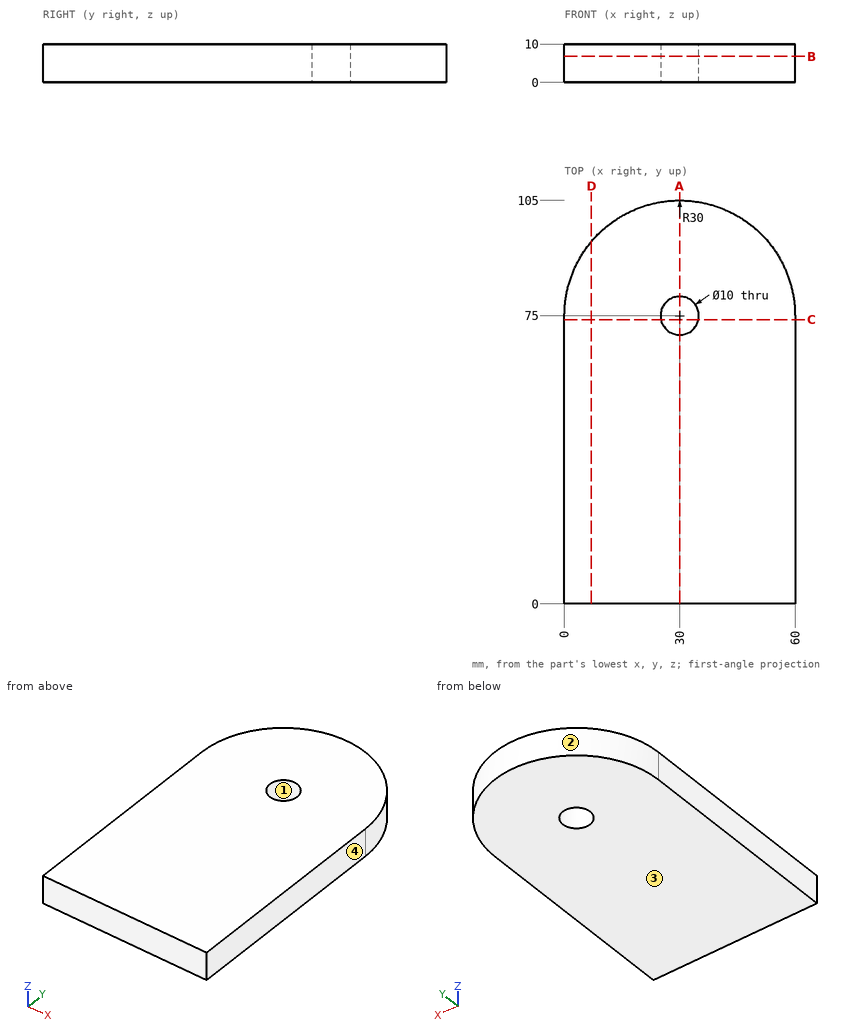
The figure shows three views and two pictorial views of one solid part (mm, origin at its lowest corner). Answer the questions. Round coordinates to 2 decimals unless told otherwise and drop trailing zeros. Loops run counter-clockwise (first coordinate to the right, second up) from the corner with the lowest first, then second, coordinate; pieces in that order, holes last. Notation, with made-up numbers: (-9, 37) - (20, 37) arc R30 ccw to (20, 61) - close; hole circle Ø11 at (-16, 60). An arc over 180 degrees is marked (long way). Use one line per item in the form item = value. Start each with the question number.
(1) Find section C-C on y = 74. Determine the outline of the cut face in (x, z).
(2) Determine the mould class of the marked faces 1, 2, 3 and 4 for opening direction X: +X half, -X half, draft (parallel to the pull), parting line (faces both ways), or undercut.
(3) Find section B-B on z = 6.75. Determine the outline of the cut face in (x, y), and give its area (3 significant figures).
(4) A flat-ended cylindrical pin translates along its axis: P1, Ø9, axis at x = 30, y = 75, coming from the +Z side. Find the tip coordinate at first contact, or state that the pin passes through.
(5) Consider line 1 (Y direction, x = 30, z = 5); line 2 (X direction, y = 76, z = 6.5); line 3 (Y direction, x = 26, z = 3.25). Determine where each line is inside the solid, lowest interval first.
(6) Find section A-A on x = 30. Determine the outline of the cut face in (y, z), and give its area (3 significant figures).
(7) Find section D-D on x = 7. Determine the outline of the cut face in (y, z).
Answer list:
q1.outline = (0, 0) - (25.1, 0) - (25.1, 10) - (0, 10) - close; (34.9, 0) - (60, 0) - (60, 10) - (34.9, 10) - close
q2.face_1 = undercut
q2.face_2 = parting line
q2.face_3 = draft
q2.face_4 = +X half
q3.outline = (0, 0) - (60, 0) - (60, 75) arc R30 ccw to (0, 75) - close; hole circle Ø10 at (30, 75)
q3.area = 5,840 mm^2
q4.P1 = through
q5.line_1 = 0 to 70, 80 to 105
q5.line_2 = 0.02 to 25.1, 34.9 to 59.98
q5.line_3 = 0 to 72, 78 to 104.73
q6.outline = (0, 0) - (70, 0) - (70, 10) - (0, 10) - close; (80, 0) - (105, 0) - (105, 10) - (80, 10) - close
q6.area = 950 mm^2
q7.outline = (0, 0) - (94.26, 0) - (94.26, 10) - (0, 10) - close
